Geometry check sheet. Reference: drawing and pictorial views, mm from the part's lowest x, y, z. A direction names the side the tool comes from. Coordinates: 2 decimals unless noted, no trailing zeros. Order: outer loops, then holes, each group sorted by start corner. A loop starts at its lowest first (then second) coordinate and runs counter-clockwise, first axis right, second up. Notation, with made-up numbers: (78, 75) -> (86, 75) arc R22 cw to (86, 87) -> close; hole circle Ø3 at (23, -3.75). An arc over 180 degrees is marked (long way). Use CSV: the item, a comma, the result in double quotes. Start each with the question number.
1) Sectioned sample at A-A on y = 32. Record the boundary of the cut face in (x, z), then the cut area to 3 significant figures.
2) Sectioned sample at C-C on z = 13. Record the boundary of the cut face in (x, y) (3 decimals).
3) Tool access check on the marked faces 1, 2 and 3. Record the directions out of +Z, -Z, +X, -X, +Y, -Y that give a thin tool (end or side, any length) a straight path to the whole face; none if there is none.
4) Go/stop test with flat-tipped pins: pin 1 (10 mm diameter, centred on x = 58, z = 18.5, fed in from -Y); pin 2 (25 mm diameter, centred on x = 55.5, y = 37, fed in from -Z); pin 3 (16 mm diameter, centred on y = 23, z = 18.5, fed in from +X) (3 decimals); pin 4 (1 mm diameter, centred on x = 29, y = 53, fed in from +Z). Record where each tip stops, or that it passes through.
5) Sectioned sample at D-D on z = 21. Record the boundary of the cut face in (x, y).
6) Sectioned sample at B-B on x = 50. Record the boundary of the cut face in (y, z).
7) Release check for a two-part mould opening along X. For the marked faces 4, 5, 6 and 7 record: released by +X, released by -X, zero draft, split by the parting line, or undercut.
8) Scan lines: line 1 along Y through (x, z) = (52, 11); line 2 along X through (y, z) = (13, 20) (3 decimals); line 3 along X through (y, z) = (21.5, 23). Record each from-to range of solid material in increasing order.
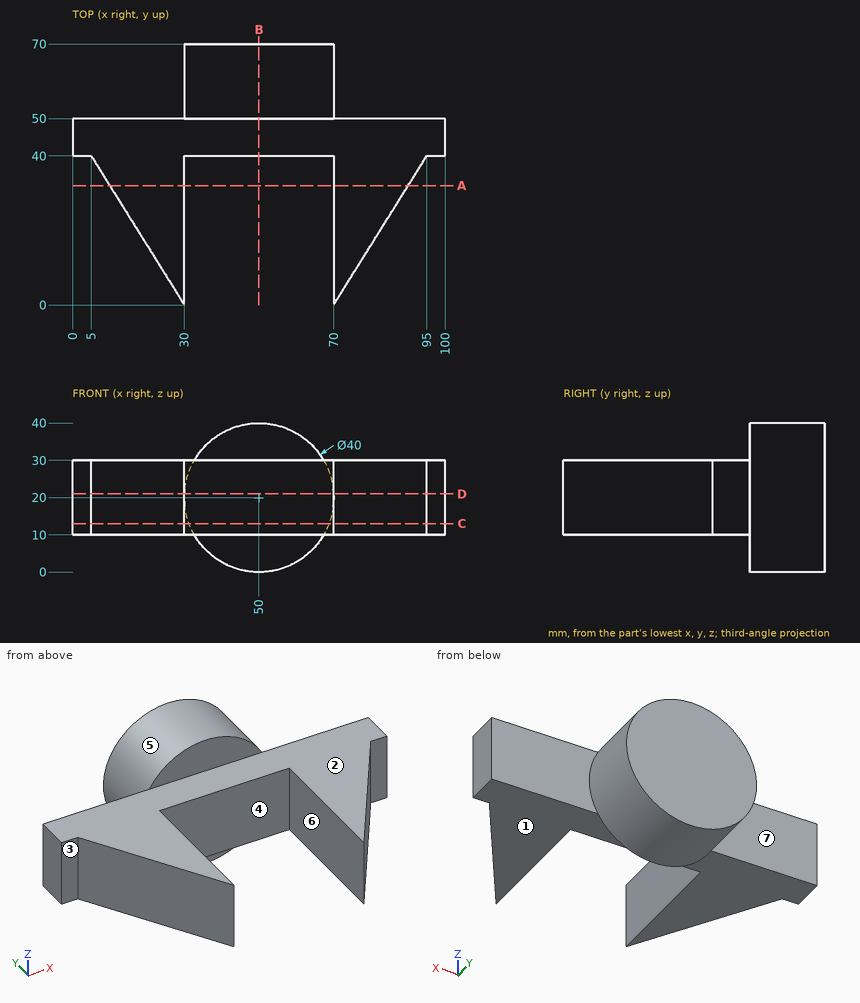
Answers follow:
1,outline,"(10, 10) -> (30, 10) -> (30, 30) -> (10, 30) -> close; (70, 10) -> (90, 10) -> (90, 30) -> (70, 30) -> close"
1,area,"800 mm²"
2,outline,"(0, 40) -> (5, 40) -> (30, 0) -> (30, 40) -> (70, 40) -> (70, 0) -> (95, 40) -> (100, 40) -> (100, 50) -> (68.735, 50) -> (68.735, 70) -> (31.265, 70) -> (31.265, 50) -> (0, 50) -> close"
3,face 1,"-Z, +X, -X, -Y"
3,face 2,"+Z, +X, -X, -Y"
3,face 3,"+Z, -Z, -X, -Y"
4,pin 1,"stops at y = 40"
4,pin 2,"stops at z = 10"
4,pin 3,"stops at x = 89.375"
4,pin 4,"passes through"
5,outline,"(0, 40) -> (5, 40) -> (30, 0) -> (30, 40) -> (70, 40) -> (70, 0) -> (95, 40) -> (100, 40) -> (100, 50) -> (69.97, 50) -> (69.97, 70) -> (30.03, 70) -> (30.03, 50) -> (0, 50) -> close"
6,outline,"(40, 10) -> (50, 10) -> (50, 0) -> (70, 0) -> (70, 40) -> (50, 40) -> (50, 30) -> (40, 30) -> close"
7,face 4,"undercut"
7,face 5,"split by the parting line"
7,face 6,"undercut"
7,face 7,"zero draft"
8,line 1,"y = 40 to 70"
8,line 2,"x = 21.875 to 30, 70 to 78.125"
8,line 3,"x = 16.56 to 30, 70 to 83.44"
